Read the model definition and answer for the solid it produces. Units are mm, in the model's axes. A direction names the side the tool comes from. Coordinates: 2 decimals unless noted, no trailing zeros. Write each loop counter-clockwise with the first axis right and the second up, starting at its lowest first coordinate (ties: lowest second). Pieces come first, ordered by that corner, then holes.
Item 1: Section A-A (y = 0) is taken. Give the vertices of the cut face in (x, z), then the cut area to 3 significant figures.
Item 2: A tool of negligible diameter and unlimited length cuts with its end or side. For faces 1 (the face through (0.5, 1, -1)), 2 (the face through (0, 0, 14.2)), from which of +Z, -Z, +X, -X, +Y, -Y can it reach the whole face along a straight path? Write none if from no direction.
Item 3: Determine the mould class of faces 3 (the face through (-1.5, 0, -1)), 4 (the face through (1, -1, -1.8)), 5 (the face through (-1.45, 0.06, 7.17)) for opening direction Y: released by +Y, released by -Y, zero draft, split by the parting line, or undercut.
Item 4: Each of these flat-tipped pins is pushed along its axis until it touches: P1, Ø1.5, axis at x = -2, z = 10.5, coming from the +Y side; P2, Ø0.5, axis at x = 1, z = -1, coming from the -Y side; P3, Ø0.5, axis at y = 1, z = -1.5, coming from the +X side; P4, Ø1.5, axis at x = -2, y = 0, coming from the +Z side. Where does it stop, or does it pass through?
Item 5: Straight lines are drawn through the part: probe 1 along X at (y, z) = (-0.6, -0.75); probe 2 along Z at (x, y) = (-1, 0.45); probe 3 along X at (y, z) = (-0.1, 12.75). For each, find the intervals that lie inside material, in ascending order.
from build123d import *

# Parameters (mm, degrees)
F0_R        = 1.45
F1_DEPTH    = 14.2
F2_R        = 2.9
F3_DEPTH    = 1.8
F4_W        = 1
F4_H        = 1
F5_DEPTH    = 1.5
F6_S5_R     = 1.45
F6_T6_DEPTH = 6


# Not quite as in the source:
# - a fillet or chamfer that OpenCascade refuses, or shapes differently, is made with other operations: its cross-section is extruded or revolved along the edge and cut away or added


with BuildPart() as f1:
    # F0 (on Top) → F1 (new body)
    with BuildSketch(Plane.XY):
        Circle(F0_R)
    extrude(amount=F1_DEPTH)

    # F2 (on Top) → F3 (join)
    with BuildSketch(Plane.XY):
        Circle(F2_R)
    extrude(amount=-F3_DEPTH)

    # F4 (on face) → F5 (cut)
    with BuildSketch(Plane(origin=(0, 0, -1.8), x_dir=(1, 0, 0), z_dir=(0, 0, -1))):
        with Locations((1, 0)):
            Rectangle(F4_W, F4_H)
        Rectangle(F4_W, F4_H)
        with Locations((0, 1)):
            Rectangle(F4_W, F4_H)
        with Locations((-1, 0)):
            Rectangle(F4_W, F4_H)
        with Locations((0, -1)):
            Rectangle(F4_W, F4_H)
    extrude(amount=-F5_DEPTH, mode=Mode.SUBTRACT)

    # F6: chamfer of 1.5 on 1 edges, made by hand


with BuildPart() as f6_tool2:
    # F6_s3 → F6_t4 (revolve)
    with BuildSketch(Plane.XZ):
        Polygon((2.9, -1.5), (1.4, 0), (2.9, 0), align=None)
    revolve(axis=Axis((0, 0, 0), (0, 0, 1)))

    # F6_s5 → F6_t6 (cut, symmetric)
    with BuildSketch(Plane.XY.offset(-0.7)):
        Circle(F6_S5_R)
    extrude(amount=F6_T6_DEPTH, both=True, mode=Mode.SUBTRACT)


with BuildPart() as f1_1:
    add(f1.part)

    # F6_t1: cut F6_tool2
    add(f6_tool2.part, mode=Mode.SUBTRACT)


solid = f1_1.part
Established:
1. outline: (-2.9, -1.8) - (-1.5, -1.8) - (-1.5, -0.3) - (1.5, -0.3) - (1.5, -1.8) - (2.9, -1.8) - (2.9, -1.5) - (1.45, -0.05) - (1.45, 14.2) - (-1.45, 14.2) - (-1.45, -0.05) - (-2.9, -1.5) - close
1. area: 44.9 mm2
2. face 1: -Z
2. face 2: +Z, +X, -X, +Y, -Y
3. face 3: undercut
3. face 4: zero draft
3. face 5: split by the parting line
4. P1: stops at y = 0.73
4. P2: stops at y = -2.47
4. P3: stops at x = 2.8
4. P4: stops at z = 14.2
5. probe 1: x = -2.06 to -0.5, 0.5 to 2.06
5. probe 2: z = -0.3 to 14.2
5. probe 3: x = -1.45 to 1.45
